from build123d import *

# Parameters (mm, degrees)
SKETCH_R     = 4.25
PAD_DEPTH    = 4
SKETCH001_R  = 1.25
PAD001_DEPTH = 4


with BuildPart() as part:
    # Sketch → Pad (new body)
    with BuildSketch(Plane.XY):
        with BuildLine():
            ThreePointArc((-14, 14), (-20, 20), (-26, 14))
            ThreePointArc((-26, 14), (-24.956276, 6.707245), (-21.908902, 0))
            Line((-21.908902, 0), (21.908902, 0))
            ThreePointArc((21.908902, 0), (24.956276, 6.707245), (26, 14))
            ThreePointArc((26, 14), (20, 20), (14, 14))
            Line((14, 5), (14, 14))
            Line((-14, 5), (14, 5))
            Line((-14, 14), (-14, 5))
        make_face()
        with Locations((-20, 14)):
            Circle(SKETCH_R, mode=Mode.SUBTRACT)
        with Locations((20, 14)):
            Circle(SKETCH_R, mode=Mode.SUBTRACT)
    extrude(amount=PAD_DEPTH)

    # Sketch001 (on Face4 of Pad) → Pad001 (join)
    with BuildSketch(Plane.XZ):
        with BuildLine():
            Line((-5.64, 7.54), (-5.64, 3.19))
            Line((-5.64, 3.19), (5.64, 3.19))
            Line((5.64, 3.19), (5.64, 7.54))
            Line((8.89, 10.79), (5.64, 7.54))
            ThreePointArc((12.14, 7.54), (11.188097, 9.838097), (8.89, 10.79))
            Line((12.14, 7.54), (12.14, 0))
            Line((12.14, 0), (-12.14, 0))
            Line((-12.14, 0), (-12.14, 7.54))
            ThreePointArc((-8.89, 10.79), (-11.188097, 9.838097), (-12.14, 7.54))
            Line((-8.89, 10.79), (-5.64, 7.54))
        make_face()
        with Locations((-8.89, 7.54)):
            Circle(SKETCH001_R, mode=Mode.SUBTRACT)
        with Locations((8.89, 7.54)):
            Circle(SKETCH001_R, mode=Mode.SUBTRACT)
    extrude(amount=-PAD001_DEPTH)


solid = part.part
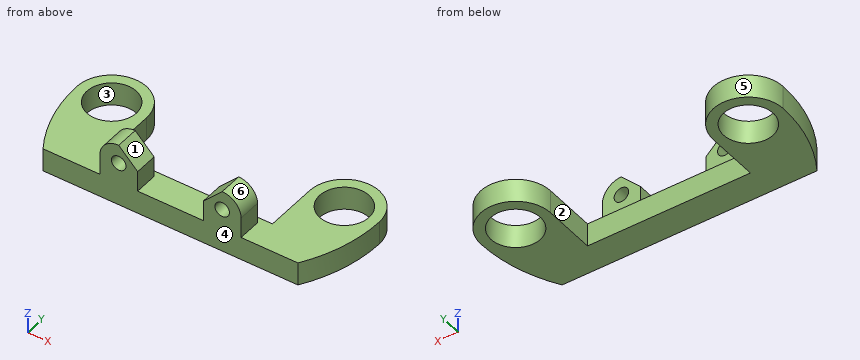
Could you check a few things on this model? Use its own coordinates, in mm. Face numbers are marked on the shaded views. A direction names the side the tool comes from. Coordinates: 2 decimals unless noted, no trailing zeros. Order: outer loops, then holes, each group sorted by start corner. A loop starts at its lowest first (then second) coordinate and runs counter-clockwise, first axis right, second up. Notation, with made-up numbers: (36, 40.5) -> (91, 40.5) arc R21 ccw to (91, 57.5) -> close; hole circle Ø4 at (52.25, 83.25). An arc over 180 degrees is marked (long way). One line per question, with ' | ' between items.
Q1. Imagine slicing it at D-D on y = 17.75. Please give me the cut outline in (x, z), and give its area (3 significant figures).
Return value:
outline: (-24.68, 0) -> (-22, 0) -> (-22, 4) -> (-24.68, 4) -> close; (-18, 0) -> (-15.32, 0) -> (-15.32, 4) -> (-18, 4) -> close; (15.32, 0) -> (18, 0) -> (18, 4) -> (15.32, 4) -> close; (22, 0) -> (24.68, 0) -> (24.68, 4) -> (22, 4) -> close | area: 42.9 mm²
Q2. If I drill on L1, parallel to Z at x = -8.89, y = 1.5; L2, parallel to Y at x = -20, z = 3.05; L3, parallel to Y at x = -5, z = 1.5, over which ranges is the centre line in solid material (lowest first)?
Return value:
L1: 0 to 6.29, 8.79 to 10.79 | L2: 0 to 9.75, 18.25 to 20 | L3: 0 to 5
Q3. Imagine slicing it at B-B on x = 20. Please give me the cut outline in (y, z).
Return value:
outline: (0, 0) -> (9.75, 0) -> (9.75, 4) -> (0, 4) -> close; (18.25, 0) -> (20, 0) -> (20, 4) -> (18.25, 4) -> close
Q4. Imagine slicing it at C-C on z = 2.75. Please give me the cut outline in (x, y).
Return value:
outline: (-26, 14) arc R26 ccw to (-21.91, 0) -> (21.91, 0) arc R26 ccw to (26, 14) arc R6 ccw to (14, 14) -> (14, 5) -> (-14, 5) -> (-14, 14) arc R6 ccw to start; hole circle Ø8.5 at (-20, 14); hole circle Ø8.5 at (20, 14)
Q5. I'm going to push flat-ended pins straight in: P1, Ø1.8, axis at y = 1.5, z = 6, coming from the -X side; P2, Ø2, axis at y = 10.5, z = 3, coming from the +X side; P3, Ø4, axis at y = 1, z = 6.5, coming from the +X side; P4, Ø6, axis at x = -4, z = 8, coming from the -Y side. Where does each tip first touch, or does it pass through?
Return value:
P1: x = -12.14 | P2: x = 25.88 | P3: x = 12.14 | P4: y = 0
Q6. On a 3-axis mill with a long thin cutter (end or side, diameter ignored), from which of +Z, -Z, +X, -X, +Y, -Y can I reach the whole of each face in a straight line? I mean the marked faces 1, 2 and 3. Say none if no direction works.
Return value:
face 1: +Z, +Y, -Y | face 2: +Z, -Z, +Y | face 3: +Z, -Z
Q7. Imagine slicing it at A-A on z = 5.25. Please give me the cut outline in (x, y), and give its area (3 significant figures).
Return value:
outline: (-12.14, 0) -> (-5.64, 0) -> (-5.64, 4) -> (-12.14, 4) -> close; (5.64, 0) -> (12.14, 0) -> (12.14, 4) -> (5.64, 4) -> close | area: 52.0 mm²
Q8. Thinking about a two-plate mould opening in X: for the marked faces 4, 5 and 6, which applies, pulls with the +X half, pulls with the -X half, needs draft (parallel to the pull), parting line crosses it, or undercut?
Return value:
face 4: needs draft | face 5: undercut | face 6: pulls with the +X half
